from build123d import *

# Parameters (mm, degrees)
SKETCH1_W           = 254
SKETCH1_H           = 38.1
SKETCH1_W_2         = 225.806
SKETCH1_H_2         = 6.604
BOSS_EXTRUDE1_DEPTH = 6.604
CUT_EXTRUDE1_DEPTH  = 7.604
FILLET1_R           = 6.35


with BuildPart() as part:
    # Sketch1 → Boss-Extrude1 (new body)
    with BuildSketch(Plane(origin=(0, 0, 0), x_dir=(1, 0, 0), z_dir=(0, 1, 0))):
        Rectangle(SKETCH1_W, SKETCH1_H)
        Rectangle(SKETCH1_W_2, SKETCH1_H_2, mode=Mode.SUBTRACT)
    extrude(amount=BOSS_EXTRUDE1_DEPTH)

    # Sketch2 → Cut-Extrude1 (cut, through all)
    with BuildSketch(Plane(origin=(0, 6.604, 0), x_dir=(1, 0, 0), z_dir=(0, 1, 0))):
        with BuildLine():
            Line((-120.65, 14.859), (-107.95, 14.859))
            ThreePointArc((-107.95, 14.859), (-105.791, 12.7), (-107.95, 10.541))
            Line((-107.95, 10.541), (-120.65, 10.541))
            ThreePointArc((-120.65, 10.541), (-122.809, 12.7), (-120.65, 14.859))
        make_face()
        with BuildLine():
            Line((-120.65, -10.541), (-107.95, -10.541))
            ThreePointArc((-107.95, -10.541), (-105.791, -12.7), (-107.95, -14.859))
            Line((-107.95, -14.859), (-120.65, -14.859))
            ThreePointArc((-120.65, -14.859), (-122.809, -12.7), (-120.65, -10.541))
        make_face()
    cut_extrude1 = extrude(amount=-CUT_EXTRUDE1_DEPTH, mode=Mode.SUBTRACT)

    # Mirror1: Cut-Extrude1 across plane
    add(cut_extrude1.mirror(Plane(origin=(0, 0, 0), x_dir=(0, 0, 1), z_dir=(1, 0, 0))), mode=Mode.SUBTRACT)

    # Fillet1
    fillet1_edges = [part.edges().sort_by_distance(p)[0] for p in [
        (-127, 3.302, -19.05),
        (127, 3.302, -19.05),
        (127, 3.302, 19.05),
        (-127, 3.302, 19.05),
    ]]
    fillet(fillet1_edges, radius=FILLET1_R)


solid = part.part
Geometry: final body of the model. Coordinates: model frame, mm. A direction names the side the tool comes from. Give positions to 0.01 mm unless a question says otherwise; leave off trailing zeros. Order: outer loops, then holes, each group sorted by start corner. A loop starts at its lowest first (then second) coordinate and runs counter-clockwise, first axis right, second up. Notation, with made-up numbers: (-20.5, 29) -> (2.5, 29) arc R23 cw to (2.5, 60) -> close; hole circle Ø5 at (13, 77.5). An arc over 180 degrees is marked (long way). Put each result on its own line as item: value.
Q1. Section C-C, the plane y = 4.5. Return loops of the section in (x, z).
Here are the results:
outline: (-127, -12.7) arc R6.35 ccw to (-120.65, -19.05) -> (120.65, -19.05) arc R6.35 ccw to (127, -12.7) -> (127, 12.7) arc R6.35 ccw to (120.65, 19.05) -> (-120.65, 19.05) arc R6.35 ccw to (-127, 12.7) -> close; hole (-120.65, -14.86) -> (-107.95, -14.86) arc R2.16 ccw to (-107.95, -10.54) -> (-120.65, -10.54) arc R2.16 ccw to start; hole (-120.65, 10.54) -> (-107.95, 10.54) arc R2.16 ccw to (-107.95, 14.86) -> (-120.65, 14.86) arc R2.16 ccw to start; hole (-112.9, -3.3) -> (112.9, -3.3) -> (112.9, 3.3) -> (-112.9, 3.3) -> close; hole (107.95, -14.86) -> (120.65, -14.86) arc R2.16 ccw to (120.65, -10.54) -> (107.95, -10.54) arc R2.16 ccw to start; hole (107.95, 10.54) -> (120.65, 10.54) arc R2.16 ccw to (120.65, 14.86) -> (107.95, 14.86) arc R2.16 ccw to start
Q2. Section A-A, the plane x = 51.5. Return loops of the section in (y, z).
Here are the results:
outline: (0, -19.05) -> (6.6, -19.05) -> (6.6, -3.3) -> (0, -3.3) -> close; (0, 3.3) -> (6.6, 3.3) -> (6.6, 19.05) -> (0, 19.05) -> close
Q3. Material intervals for L1, parallel to Z at x = -109, y = 2.25; L2, parallel to Z at x = -70, y = 3.25; L3, parallel to X at y = 4.75, z = 12.5, sorted ascending.
Here are the results:
L1: z = -19.05 to -14.86, -10.54 to -3.3, 3.3 to 10.54, 14.86 to 19.05
L2: z = -19.05 to -3.3, 3.3 to 19.05
L3: x = -127 to -122.8, -105.8 to 105.8, 122.8 to 127
Q4. Reachability of faces 1 (the face through (105.79, 3.35, 12.65)), 2 (the face through (-127, 3, 0)) from +Z, -Z, +X, -X, +Y, -Y: full face, straight path, thin tool, end or side. Return the list, or none.
Here are the results:
face 1: +Y, -Y
face 2: +Z, -Z, -X, +Y, -Y
Q5. Section B-B, the plane z = -0.5. Return loops of the section in (x, y).
Here are the results:
outline: (-127, 0) -> (-112.9, 0) -> (-112.9, 6.6) -> (-127, 6.6) -> close; (112.9, 0) -> (127, 0) -> (127, 6.6) -> (112.9, 6.6) -> close
Q6. Draft query along Z for faces 3 (the face through (127, 3, 0)), 4 (the face through (125.09, 3.35, -17.24)), 5 (the face through (-2, 3, -3.302)). Return one class per face: released by +Z, released by -Z, zero draft, split by the parting line, or undercut.
Here are the results:
face 3: zero draft
face 4: released by -Z
face 5: undercut
